Read the model definition and answer for the solid it produces. Units are mm, in the model's axes. A direction names the side the tool comes from. Coordinates: 2 decimals unless noted, no trailing zeros. Loops run counter-clockwise (first coordinate to the right, second up) from the corner with the lowest first, then second, coordinate; pieces in that order, holes last.
Q1. Straight lines are drawn through the part: line 1 (Y direction, x = 0, z = -6); line 2 (Z direction, x = 3, y = 6.5); line 3 (X direction, y = 0.5, z = -6.5). For each, find the intervals that lie inside material, in ascending order.
Q2. Flat-ended cylindrical pins translate along their axes: P1, Ø5, axis at y = 0, z = -6, coming from the -X side; P2, Ø4, axis at y = -4, z = -4.5, coming from the -X side; P3, Ø4, axis at x = 4.5, z = -6, coming from the +Y side. Find the tip coordinate at first contact, or state that the pin passes through.
Q3. Section C-C (z = -3.75) is taken. Give the vertices of the cut face in (x, y), then the cut area to 3 significant figures.
Q4. The mould has two halves that part along Y. Classify faces 3 (the face through (1.476, 2.837, -5.931)), 4 (the face through (-2, 2, -11.001)), 5 (the face through (2.385, -0.751, -5.423)): pulls with the +Y half, pulls with the -Y half, needs draft (parallel to the pull), parting line crosses it, or undercut.
Q5. Which of the six approach directions +Z, -Z, +X, -X, +Y, -Y give full straight-line access (tool end or side, diameter ignored) to faces 1 (the face through (4, 0, -1.001)), 2 (the face through (2, 2, 0))?
Q6. Section D-D (x = -7) is taken. Give the vertices of the cut face in (y, z), then the cut area to 3 significant figures.
Q7. Section A-A (y = 0) is taken. Give the vertices of the cut face in (x, z).
from build123d import *

# Parameters (mm, degrees)
SKETCH2_W           = 1.00076
SKETCH2_H           = 9.4996
SKETCH3_R           = 2.50000008
CUT_EXTRUDE1_DEPTH  = 2.54
SKETCH4_R           = 3.19786
SKETCH4_R_2         = 2.50000008
BOSS_EXTRUDE1_DEPTH = 9.99998


with BuildPart() as part:
    # Sketch2 → Revolve1 (revolve)
    with BuildSketch(Plane(origin=(0, 0, 0), x_dir=(0, 0, -1), z_dir=(1, 0, 0)), mode=Mode.PRIVATE) as revolve1_sk:
        with Locations((0.50038, 4.7498)):
            Rectangle(SKETCH2_W, SKETCH2_H)
    revolve(revolve1_sk.sketch.rotate(Axis((0, 0, -1.00076), (0, 0, 1)), 90), axis=Axis((0, 0, -1.00076), (0, 0, 1)))

    # Sketch3 → Cut-Extrude1 (cut)
    with BuildSketch(Plane.XY):
        Circle(SKETCH3_R)
    extrude(amount=-CUT_EXTRUDE1_DEPTH, mode=Mode.SUBTRACT)

    # Sketch4 → Boss-Extrude1 (add)
    with BuildSketch(Plane(origin=(0, 0, -1.00076), x_dir=(-1, 0, 0), z_dir=(0, 0, -1))):
        with Locations(Location((0, 0, 0), (0, 0, 180))):
            Circle(SKETCH4_R)
        with Locations(Location((0, 0, 0), (0, 0, 180))):
            Circle(SKETCH4_R_2, mode=Mode.SUBTRACT)
    extrude(amount=BOSS_EXTRUDE1_DEPTH)


solid = part.part
Numbers:
1. line 1: y = -3.2 to -2.5, 2.5 to 3.2
1. line 2: z = -1 to 0
1. line 3: x = -3.16 to -2.45, 2.45 to 3.16
2. P1: stops at x = -3.2
2. P2: stops at x = -2.5
2. P3: stops at y = 1.99
3. outline: circle Ø6.4 at (0, 0); hole circle Ø5 at (0, 0)
3. area: 12.5 mm2
4. face 3: parting line crosses it
4. face 4: needs draft
4. face 5: undercut
5. face 1: -Z
5. face 2: +Z, +X, -X, +Y, -Y
6. outline: (-6.42, -1) - (6.42, -1) - (6.42, 0) - (-6.42, 0) - close
6. area: 12.9 mm2
7. outline: (-9.5, -1) - (-3.2, -1) - (-3.2, -11) - (-2.5, -11) - (-2.5, 0) - (-9.5, 0) - close; (2.5, -11) - (3.2, -11) - (3.2, -1) - (9.5, -1) - (9.5, 0) - (2.5, 0) - close
